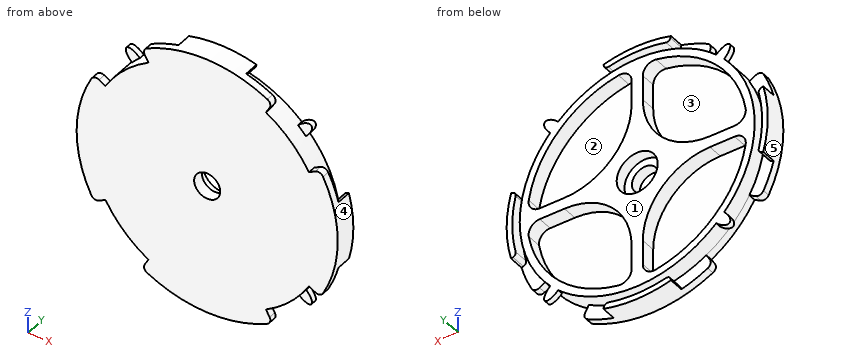
from build123d import *

# Parameters (mm, degrees)
SKETCH1_R                                           = 35
BOSS_EXTRUDE1_DEPTH                                 = 2
SKETCH2_R                                           = 31.5
BOSS_EXTRUDE2_DEPTH                                 = 4
SKETCH4_R                                           = 35
SKETCH4_R_2                                         = 33.5
BOSS_EXTRUDE3_DEPTH                                 = 4
CUT_EXTRUDE2_START                                  = -6
CUT_EXTRUDE2_DEPTH                                  = 6
CUT_EXTRUDE3_START                                  = -4
CUT_EXTRUDE3_DEPTH                                  = 4
SKETCH7_RX                                          = 3.5
SKETCH7_RY                                          = 1.5
BOSS_EXTRUDE4_DEPTH                                 = 1.5
CUT_EXTRUDE1_DEPTH                                  = 4
FILLET1_R                                           = 18
FILLET2_R                                           = 3
FILLET3_R                                           = 1.5
FILLET4_R                                           = 1
CIRPATTERN1_COUNT                                   = 4
FILLET1_OF_CIRPATTERN1_R                            = 18
FILLET2_OF_CIRPATTERN1_R                            = 3
FILLET3_OF_CIRPATTERN1_R                            = 1.5
FILLET4_OF_CIRPATTERN1_R                            = 1
CBORE_FOR_M6_HEX_SOCKET_HEAD_CAP_SCREW1_D           = 7
CBORE_FOR_M6_HEX_SOCKET_HEAD_CAP_SCREW1_CBORE_D     = 11
CBORE_FOR_M6_HEX_SOCKET_HEAD_CAP_SCREW1_CBORE_DEPTH = 3


# Read off the part's stored shape, not the designer's step: Cut-Extrude2
with BuildPart() as part:
    # Sketch1 → Boss-Extrude1 (new body)
    with BuildSketch(Plane(origin=(0, 0, 0), x_dir=(1, 0, 0), z_dir=(0, 1, 0))):
        with Locations(Location((0, 0, 0), (0, 0, 270))):
            Circle(SKETCH1_R)
    extrude(amount=BOSS_EXTRUDE1_DEPTH)

    # Sketch2 → Boss-Extrude2 (add)
    with BuildSketch(Plane(origin=(0, 2, 0), x_dir=(1, 0, 0), z_dir=(0, 1, 0))):
        with Locations(Location((0, 0, 0), (0, 0, 270))):
            Circle(SKETCH2_R)
    extrude(amount=BOSS_EXTRUDE2_DEPTH)

    # Sketch4 → Boss-Extrude3 (add)
    with BuildSketch(Plane(origin=(0, 2, 0), x_dir=(1, 0, 0), z_dir=(0, 1, 0))):
        with Locations(Location((0, 0, 0), (0, 0, 270))):
            Circle(SKETCH4_R)
        with Locations(Location((0, 0, 0), (0, 0, 270))):
            Circle(SKETCH4_R_2, mode=Mode.SUBTRACT)
    extrude(amount=BOSS_EXTRUDE3_DEPTH)

    # Cut-Extrude2 outline → Cut-Extrude2 (cut)
    with BuildSketch(Plane(origin=(0, 6, 0), x_dir=(1, 0, 0), z_dir=(0, 1, 0)).offset(CUT_EXTRUDE2_START)):
        with BuildLine():
            ThreePointArc((30.310889132, 17.5), (24.748737342, 24.748737342), (17.5, 30.310889132))
            Line((17.5, 30.310889132), (15.75, 27.279800219))
            ThreePointArc((15.75, 27.279800219), (22.273863607, 22.273863607), (27.279800219, 15.75))
            Line((27.279800219, 15.75), (30.310889132, 17.5))
        make_face()
    cut_extrude2 = extrude(amount=CUT_EXTRUDE2_DEPTH, mode=Mode.SUBTRACT)

    # Sketch6 → Cut-Extrude3 (cut)
    with BuildSketch(Plane(origin=(0, 6, 0), x_dir=(1, 0, 0), z_dir=(0, 1, 0)).offset(CUT_EXTRUDE3_START)):
        with BuildLine():
            Line((8.152799921, 30.426663528), (9.058666579, 33.80740392))
            ThreePointArc((9.058666579, 33.80740392), (24.748737342, 24.748737342), (33.80740392, 9.058666579))
            Line((33.80740392, 9.058666579), (30.426663528, 8.152799921))
            ThreePointArc((30.426663528, 8.152799921), (22.273863607, 22.273863607), (8.152799921, 30.426663528))
        make_face()
    cut_extrude3 = extrude(amount=CUT_EXTRUDE3_DEPTH, mode=Mode.SUBTRACT)

    # Sketch7 → Boss-Extrude4 (add)
    with BuildSketch(Plane(origin=(0, 6, 0), x_dir=(1, 0, 0), z_dir=(0, 1, 0))):
        with Locations(Location((22.273863607, 22.273863607), (0, 0, 45))):
            Ellipse(SKETCH7_RX, SKETCH7_RY)
    boss_extrude4 = extrude(amount=-BOSS_EXTRUDE4_DEPTH)

    # Sketch3 → Cut-Extrude1 (cut)
    with BuildSketch(Plane(origin=(0, 6, 0), x_dir=(1, 0, 0), z_dir=(0, 1, 0))):
        with BuildLine():
            Line((1.5, 1.5), (1.5, 29.461839725))
            ThreePointArc((1.5, 29.461839725), (20.859650045, 20.859650045), (29.461839725, 1.5))
            Line((29.461839725, 1.5), (1.5, 1.5))
        make_face()
    cut_extrude1 = extrude(amount=-CUT_EXTRUDE1_DEPTH, mode=Mode.SUBTRACT)

    # Fillet1
    fillet1_edges = [part.edges().sort_by_distance(p)[0] for p in [
        (1.5, 4, -1.5),
    ]]
    fillet(fillet1_edges, radius=FILLET1_R)

    # Fillet2
    fillet2_edges = [part.edges().sort_by_distance(p)[0] for p in [
        (29.461839725, 4, -1.5),
        (1.5, 4, -29.461839725),
    ]]
    fillet(fillet2_edges, radius=FILLET2_R)

    # Fillet3
    fillet3_edges = [part.edges().sort_by_distance(p)[0] for p in [
        (17.5, 1, -30.310889132),
        (30.310889132, 1, -17.5),
    ]]
    fillet(fillet3_edges, radius=FILLET3_R)

    # Fillet4
    fillet4_edges = [part.edges().sort_by_distance(p)[0] for p in [
        (8.670438011, 4, -32.358515181),
        (32.358515181, 4, -8.670438011),
    ]]
    fillet(fillet4_edges, radius=FILLET4_R)

    # CirPattern1: Cut-Extrude2, Cut-Extrude3, Boss-Extrude4, Cut-Extrude1 ×4 about axis
    cirpattern1_axis = Axis((0, 6, 0), (0, -1, 0))
    add([cut_extrude2.rotate(cirpattern1_axis, i * 360 / CIRPATTERN1_COUNT) for i in range(1, CIRPATTERN1_COUNT)], mode=Mode.SUBTRACT)
    add([cut_extrude3.rotate(cirpattern1_axis, i * 360 / CIRPATTERN1_COUNT) for i in range(1, CIRPATTERN1_COUNT)], mode=Mode.SUBTRACT)
    add([boss_extrude4.rotate(cirpattern1_axis, i * 360 / CIRPATTERN1_COUNT) for i in range(1, CIRPATTERN1_COUNT)])
    add([cut_extrude1.rotate(cirpattern1_axis, i * 360 / CIRPATTERN1_COUNT) for i in range(1, CIRPATTERN1_COUNT)], mode=Mode.SUBTRACT)

    # Fillet1 of CirPattern1
    fillet1_of_cirpattern1_edges = [part.edges().sort_by_distance(p)[0] for p in [
        (1.5, 4, 1.5),
        (-1.5, 4, 1.5),
        (-1.5, 4, -1.5),
    ]]
    fillet(fillet1_of_cirpattern1_edges, radius=FILLET1_OF_CIRPATTERN1_R)

    # Fillet2 of CirPattern1
    fillet2_of_cirpattern1_edges = [part.edges().sort_by_distance(p)[0] for p in [
        (1.5, 4, 29.461839725),
        (29.461839725, 4, 1.5),
        (-29.461839725, 4, 1.5),
        (-1.5, 4, 29.461839725),
        (-1.5, 4, -29.461839725),
        (-29.461839725, 4, -1.5),
    ]]
    fillet(fillet2_of_cirpattern1_edges, radius=FILLET2_OF_CIRPATTERN1_R)

    # Fillet3 of CirPattern1
    fillet3_of_cirpattern1_edges = [part.edges().sort_by_distance(p)[0] for p in [
        (30.310889132, 1, 17.5),
        (17.5, 1, 30.310889132),
        (-17.5, 1, 30.310889132),
        (-30.310889132, 1, 17.5),
        (-30.310889132, 1, -17.5),
        (-17.5, 1, -30.310889132),
    ]]
    fillet(fillet3_of_cirpattern1_edges, radius=FILLET3_OF_CIRPATTERN1_R)

    # Fillet4 of CirPattern1
    fillet4_of_cirpattern1_edges = [part.edges().sort_by_distance(p)[0] for p in [
        (32.358515181, 4, 8.670438011),
        (8.670438011, 4, 32.358515181),
        (-8.670438011, 4, 32.358515181),
        (-32.358515181, 4, 8.670438011),
        (-32.358515181, 4, -8.670438011),
        (-8.670438011, 4, -32.358515181),
    ]]
    fillet(fillet4_of_cirpattern1_edges, radius=FILLET4_OF_CIRPATTERN1_R)

    # CBORE for M6 Hex Socket Head Cap Screw1 (through all)
    with Locations(Plane(origin=(0, 6, 0), x_dir=(1, 0, 0), z_dir=(0, 1, 0))):
        with Locations((0, 0)):
            CounterBoreHole(CBORE_FOR_M6_HEX_SOCKET_HEAD_CAP_SCREW1_D / 2, CBORE_FOR_M6_HEX_SOCKET_HEAD_CAP_SCREW1_CBORE_D / 2, CBORE_FOR_M6_HEX_SOCKET_HEAD_CAP_SCREW1_CBORE_DEPTH)


solid = part.part
Input: part model. Units: mm. Frame: model coordinates. Face numbers are marked on the shaded views. A direction names the side the tool comes from. Coordinates: 2 decimals unless noted, no trailing zeros. Order: outer loops, then holes, each group sorted by start corner. A loop starts at its lowest first (then second) coordinate and runs counter-clockwise, first axis right, second up. Notation, with made-up numbers: M 35.5,-26 L 52.5,-26 A25 ccw 52.5,-7 Z; hole C -28,-14 d11. An arc over 180 degrees is marked long. Write item = value, one per line. Start each with the question number.
(1) First-contact query: P1, Ø4, axis at x = 22.5, z = 23, coming from the -Y side; P2, Ø2, axis at y = 3, z = 23.5, coming from the -X side; P3, Ø3, axis at x = 2.5, y = 2.5, coming from the +Z side; P4, Ø1.5, axis at y = 3, z = 17, coming from the +X side. Flat tips, straight axial feed; report the tip coordinate or a pass-through.
(2) Section D-D on z = 18.5. Output: boundary loops of the cut face in (x, y), and give its area (3 significant figures).
(3) Section C-C on x = -11. Output: boundary loops of the cut face in (y, z), and give its area (3 significant figures).
(4) Section B-B on z = 0. Output: boundary loops of the cut face in (x, y).
(5) Section A-A on x = 0. Output: boundary loops of the cut face in (y, z).
(6) Line query: line 1 along Z through (x, y) = (0, 4.45); line 2 along X through (y, z) = (4, -22.5); line 3 along Z through (x, y) = (-4, 4.75) (1 decimal). Output: solid intervals per line, ascending. Write a range as [from, to].
(7) Reachability of the marked faces 1 and 2 from +Z, -Z, +X, -X, +Y, -Y: full face, straight path, thin tool, end or side. Return the list, or none.
(8) Pull-direction query (X, two-part tool) for the marked faces 3, 4 and 5; classes: released by +X, released by -X, zero draft, split by the parting line, or undercut.
Result set:
q1.P1 = 0
q1.P2 = -22.05
q1.P3 = 34.99
q1.P4 = 26.98
q2.outline = M -25.5,0 L 25.5,0 L 25.5,6 L 22.98,6 L 22.98,2 L 1.53,2 L 1.53,6 L -1.53,6 L -1.53,2 L -22.98,2 L -22.98,6 L -25.5,6 Z
q2.area = 134 mm²
q3.outline = M 0,-33.23 L 2,-33.23 L 2,-29.52 L 6,-29.52 L 6,-27.37 L 2,-27.37 L 2,-3.63 L 6,-3.63 L 6,3.63 L 2,3.63 L 2,27.37 L 6,27.37 L 6,29.52 L 2,29.52 L 2,33.23 L 0,33.23 Z
q3.area = 179 mm²
q4.outline = M -35,0 L -3.5,0 L -3.5,3 L -5.5,3 L -5.5,6 L -31.5,6 L -31.5,2 L -33.5,2 L -33.5,6 L -35,6 Z; M 3.5,0 L 35,0 L 35,6 L 33.5,6 L 33.5,2 L 31.5,2 L 31.5,6 L 5.5,6 L 5.5,3 L 3.5,3 Z
q5.outline = M 0,-35 L 6,-35 L 6,-33.5 L 2,-33.5 L 2,-31.5 L 6,-31.5 L 6,-5.5 L 3,-5.5 L 3,-3.5 L 0,-3.5 Z; M 0,3.5 L 3,3.5 L 3,5.5 L 6,5.5 L 6,31.5 L 2,31.5 L 2,33.5 L 6,33.5 L 6,35 L 0,35 Z
q6.line_1 = [-35, -33.5], [-31.5, -5.5], [5.5, 31.5], [33.5, 35]
q6.line_2 = [-22.05, -19.08], [-1.5, 1.5], [19.08, 22.05]
q6.line_3 = [-34.8, -33.3], [-31.2, -29.1], [-10.3, -3.8], [3.8, 10.3], [29.1, 31.2], [33.3, 34.8]
q7.face_1 = +Z, -Z, +X, -X, +Y
q7.face_2 = +Y
q8.face_3 = undercut
q8.face_4 = released by +X
q8.face_5 = released by -X
